The listing builds one solid part. Answer for the finished solid, in the listing's coordinates (mm). A direction names the side the tool comes from. Give positions to 0.01 mm unless a question says otherwise; leave off trailing zeros. Write each loop counter-clockwise with the first axis right and the second up, starting at its lowest first coordinate (ties: lowest second). Pieces come first, ordered by that corner, then holes. Notation, with made-up numbers: M -9,43 L 47,43 A28 ccw 47,62 Z; hole C 57,38 d10. An arc over 180 degrees is marked long. Return JSON: item names as keys, results as strings.
from build123d import *

# Parameters (mm, degrees)
F1_DEPTH  = 60
F2_R      = 15
F3_DEPTH  = 1.3
F3_FACE_R = 15
F4_DEPTH  = 55


with BuildPart() as f1:
    # F0 (on Top) → F1 (new body)
    with BuildSketch(Plane.XY):
        with BuildLine():
            Line((25, 30), (-25, 30))
            ThreePointArc((-25, 30), (-28.535534, 28.535534), (-30, 25))
            Line((-30, 25), (-30, -25))
            ThreePointArc((-30, -25), (-28.535534, -28.535534), (-25, -30))
            Line((-25, -30), (25, -30))
            ThreePointArc((25, -30), (28.535534, -28.535534), (30, -25))
            Line((30, -25), (30, 25))
            ThreePointArc((30, 25), (28.535534, 28.535534), (25, 30))
        make_face()
    extrude(amount=F1_DEPTH)

    # F2 (on face) → F3 (cut)
    with BuildSketch(Plane.XY.offset(60)):
        with BuildLine():
            Line((20, 25), (-20, 25))
            ThreePointArc((-20, 25), (-23.535534, 23.535534), (-25, 20))
            Line((-25, 20), (-25, -20))
            ThreePointArc((-25, -20), (-23.535534, -23.535534), (-20, -25))
            Line((-20, -25), (20, -25))
            ThreePointArc((20, -25), (23.535534, -23.535534), (25, -20))
            Line((25, -20), (25, 20))
            ThreePointArc((25, 20), (23.535534, 23.535534), (20, 25))
        make_face()
        Circle(F2_R, mode=Mode.SUBTRACT)
    extrude(amount=-F3_DEPTH, mode=Mode.SUBTRACT)

    # F3_face (on face) → F4 (cut)
    with BuildSketch(Plane.XY.offset(60)):
        Circle(F3_FACE_R)
    extrude(amount=-F4_DEPTH, mode=Mode.SUBTRACT)


solid = f1.part
Item 1: Determine the mould class of faces 3 (the flat face through (0, -30, 30)), 4 (the flat face through (0, 0, 0)), 5 (the flat face through (11, -11, 58.7)) for opening direction Y: +Y half, -Y half, draft (parallel to the pull), parting line (faces both ways), or undercut.
Geometry results:
{"face 3": "-Y half", "face 4": "draft", "face 5": "undercut"}
Item 2: Find the intervals of material crossed by line 1 (Y direction, x = 0, z = 47); line 2 (Z direction, x = 10.5, y = 9); line 3 (Y direction, x = 3, z = 25), in increasing order.
Geometry results:
{"line 1": "y = -30 to -15, 15 to 30", "line 2": "z = 0 to 5", "line 3": "y = -30 to -14.7, 14.7 to 30"}
Item 3: A cutting plane is placed at B-B, the plane z = 40. Write down the section's boundary in (x, y).
Geometry results:
{"outline": "M -30,-25 A5 ccw -25,-30 L 25,-30 A5 ccw 30,-25 L 30,25 A5 ccw 25,30 L -25,30 A5 ccw -30,25 Z; hole C 0,0 d30"}
Item 4: A cutting plane is placed at C-C, the plane y = -4.5. Write down the section's boundary in (x, z).
Geometry results:
{"outline": "M -30,0 L 30,0 L 30,60 L 25,60 L 25,58.7 L 14.31,58.7 L 14.31,5 L -14.31,5 L -14.31,58.7 L -25,58.7 L -25,60 L -30,60 Z"}
Item 5: A cutting plane is placed at A-A, the plane x = 0. Write down the section's boundary in (y, z), plus the area to 3 significant figures.
Geometry results:
{"outline": "M -30,0 L 30,0 L 30,60 L 25,60 L 25,58.7 L 15,58.7 L 15,5 L -15,5 L -15,58.7 L -25,58.7 L -25,60 L -30,60 Z", "area": "1,920 mm2"}
Item 6: A cutting plane is placed at D-D, the plane y = -22.5. Write down the section's boundary in (x, z), plus the area to 3 significant figures.
Geometry results:
{"outline": "M -30,0 L 30,0 L 30,60 L 24.33,60 L 24.33,58.7 L -24.33,58.7 L -24.33,60 L -30,60 Z", "area": "3,540 mm2"}
Item 7: Which of the six approach directions +Z, -Z, +X, -X, +Y, -Y give full straight-line access (tool end or side, diameter ignored) to faces 1 (the cylindrical face through (-24, -23, 59)), 2 (the cylindrical face through (28, -29, 30))?
Geometry results:
{"face 1": "+Z", "face 2": "+Z, -Z, +X, -Y"}
Item 8: Given pin 1 Ø18 at (x, y) = (0, 0) entering from +Z, flat-ended and moving along its own axis, determine where the tip first touches the part or whether it passes through.
Geometry results:
{"pin 1": "stops at z = 5"}
